Could you check a few things on this model? Use its own coordinates, in mm. Coordinates: 2 decimals unless noted, no trailing zeros. Write each loop counter-clockwise with the first axis right and the second up, starting at its lowest first coordinate (ties: lowest second). Pieces come first, ordered by that corner, then holes.
Item 1: I want a section at C-C on y = 1455. Please give me the cut outline in (x, z).
Item 2: If I drill on probe 1 along Y at (x, z) = (-6, 35); probe 2 along Y at (x, z) = (-85, 26); probe 3 along Y at (x, z) = (-43, 57), over which ranges is the centre line in solid material (lowest first)?
Item 3: I want a section at D-D on z = 35. State how many separate pieces and enclosed holes the cut face has, then the cut area to 3 significant figures.
Item 4: I want a section at A-A on y = 336.5. Please give me the cut outline in (x, z) (3 decimals), then the cut area to 3 significant figures.
Item 5: For P1, Ø2, axis at y = 452, z = 51.5, coming from the -X side; P2, Ø19, axis at y = 77, z = 40.5, coming from the +X side; P3, Ø3, axis at x = 50, z = 22, coming from the -Y side, each with a flat end and sliding along its axis, tell me the tip position at first contact or that it passes through.
Item 6: I want a section at B-B on x = -85. Please give me the cut outline in (y, z), then the cut area to 3 significant figures.
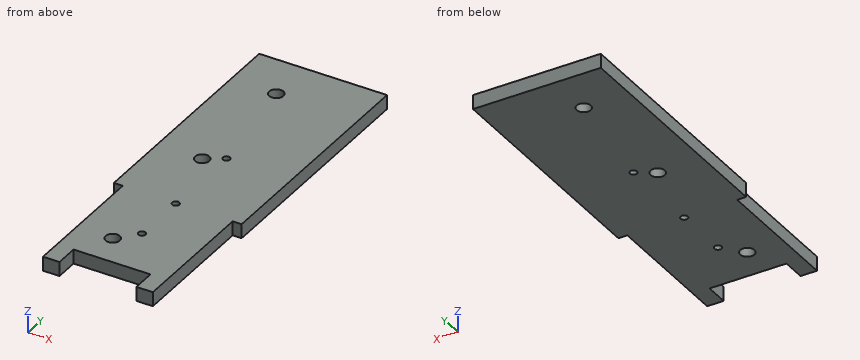
from build123d import *

# Parameters (mm, degrees)
BOSS_EXTRUDE1_DEPTH = 63.5
SKETCH2_W           = 343
SKETCH2_H           = 104
CUT_EXTRUDE1_DEPTH  = 1691.408900237
SKETCH3_R           = 31.75
CUT_EXTRUDE2_DEPTH  = 1691.408900237
SKETCH4_R           = 31.75
CUT_EXTRUDE3_DEPTH  = 1691.408900237
SKETCH5_R           = 15.875
CUT_EXTRUDE4_DEPTH  = 1691.408900237


with BuildPart() as part:
    # Sketch1 → Boss-Extrude1 (new body)
    with BuildSketch(Plane.XY):
        Polygon((-245, 0), (245, 0), (245, 590), (285, 590), (285, 1665), (-285, 1665), (-285, 590), (-245, 590), align=None)
    extrude(amount=BOSS_EXTRUDE1_DEPTH)

    # Sketch2 → Cut-Extrude1 (cut, through all)
    with BuildSketch(Plane(origin=(0, 0, 0), x_dir=(-1, 0, 0), z_dir=(0, 0, -1))):
        with Locations((0, 52)):
            Rectangle(SKETCH2_W, SKETCH2_H)
    extrude(amount=-CUT_EXTRUDE1_DEPTH, mode=Mode.SUBTRACT)

    # Sketch3 → Cut-Extrude2 (cut, through all)
    with BuildSketch(Plane.XY.offset(63.5)):
        with Locations((-82, 1455)):
            Circle(SKETCH3_R)
    extrude(amount=-CUT_EXTRUDE2_DEPTH, mode=Mode.SUBTRACT)

    # Sketch4 → Cut-Extrude3 (cut, through all)
    with BuildSketch(Plane.XY.offset(63.5)):
        with Locations((-85, 250)):
            Circle(SKETCH4_R)
        with Locations((-85, 911.9875)):
            Circle(SKETCH4_R)
    extrude(amount=-CUT_EXTRUDE3_DEPTH, mode=Mode.SUBTRACT)

    # Sketch5 → Cut-Extrude4 (cut, through all)
    with BuildSketch(Plane.XY.offset(63.5)):
        with Locations((-6.4, 336.5)):
            Circle(SKETCH5_R)
        with Locations((-6.4, 586.5)):
            Circle(SKETCH5_R)
        with Locations((-6.4, 961.5)):
            Circle(SKETCH5_R)
    extrude(amount=-CUT_EXTRUDE4_DEPTH, mode=Mode.SUBTRACT)


solid = part.part
Response values:
1. outline: (-285, 0) - (-113.75, 0) - (-113.75, 63.5) - (-285, 63.5) - close; (-50.25, 0) - (285, 0) - (285, 63.5) - (-50.25, 63.5) - close
2. probe 1: y = 104 to 320.63, 352.37 to 570.63, 602.37 to 945.63, 977.37 to 1665
2. probe 2: y = 104 to 218.25, 281.75 to 880.24, 943.74 to 1423.39, 1486.61 to 1665
2. probe 3: y = 104 to 1665
3. separate pieces: 1
3. enclosed holes: 6
3. area: 854,000 mm2
4. outline: (-245, 0) - (-22.275, 0) - (-22.275, 63.5) - (-245, 63.5) - close; (9.475, 0) - (245, 0) - (245, 63.5) - (9.475, 63.5) - close
4. area: 29,100 mm2
5. P1: stops at x = -245
5. P2: stops at x = 245
5. P3: stops at y = 104
6. outline: (104, 0) - (218.25, 0) - (218.25, 63.5) - (104, 63.5) - close; (281.75, 0) - (880.24, 0) - (880.24, 63.5) - (281.75, 63.5) - close; (943.74, 0) - (1423.39, 0) - (1423.39, 63.5) - (943.74, 63.5) - close; (1486.61, 0) - (1665, 0) - (1665, 63.5) - (1486.61, 63.5) - close
6. area: 87,000 mm2
